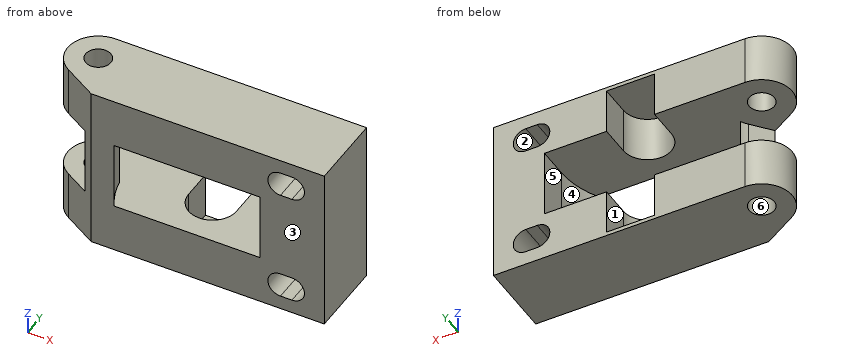
```python
from build123d import *

# Parameters (mm, degrees)
SKETCH1_R               = 1.65
BOSS_EXTRUDE1_DEPTH     = 22
CUT_EXTRUDE1_DEPTH      = 4.5
CUT_EXTRUDE1_DEPTH_BACK = 4.5
CUT_EXTRUDE3_DEPTH      = 10.5
CUT_EXTRUDE3_DEPTH_BACK = 10.5
CUT_EXTRUDE2_DEPTH      = 31.740852298


with BuildPart() as part:
    # Sketch1 → Boss-Extrude1 (new body)
    with BuildSketch(Plane.XY):
        with BuildLine():
            Line((-17, -3.464101615), (-12.607695155, -6))
            Line((-12.607695155, -6), (18, -6))
            Line((18, -6), (18, 4))
            Line((18, 4), (-15, 4))
            ThreePointArc((-15, 4), (-18.863703305, 1.03527618), (-17, -3.464101615))
        make_face()
        with Locations((-15, 0)):
            Circle(SKETCH1_R, mode=Mode.SUBTRACT)
    extrude(amount=BOSS_EXTRUDE1_DEPTH)

    # Sketch2 → Cut-Extrude1 (cut, two sides: drawn at the far end of the back side and taken through both)
    with BuildSketch(Plane.XY.offset(11).offset(-CUT_EXTRUDE1_DEPTH_BACK)):
        with BuildLine():
            Line((-11.706008895, -2.763986722), (-19.3, -11.814152904))
            Line((-19.3, -11.814152904), (-19.3, 11.3))
            Line((-19.3, 11.3), (11.3, 11.3))
            Line((11.3, 11.3), (11.3, 0))
            ThreePointArc((11.3, 0), (0.950789146, -11.259928952), (-11.14, -1.894835085))
            ThreePointArc((-11.14, -1.894835085), (-11.396702437, -2.346539297), (-11.706008895, -2.763986722))
        make_face()
    extrude(amount=CUT_EXTRUDE1_DEPTH + CUT_EXTRUDE1_DEPTH_BACK, mode=Mode.SUBTRACT)

    # Sketch4 → Cut-Extrude3 (cut, two sides: drawn at the far end of the back side and taken through both)
    with BuildSketch(Plane.XY.offset(11).offset(-CUT_EXTRUDE3_DEPTH_BACK)):
        with BuildLine():
            Line((-3.15, 0), (-3.15, 6.453034263))
            Line((-3.15, 6.453034263), (3.15, 6.453034263))
            Line((3.15, 6.453034263), (3.15, 0))
            ThreePointArc((3.15, 0), (0, -3.15), (-3.15, 0))
        make_face()
    extrude(amount=CUT_EXTRUDE3_DEPTH + CUT_EXTRUDE3_DEPTH_BACK, mode=Mode.SUBTRACT)

    # Sketch3 → Cut-Extrude2 (cut, through all)
    with BuildSketch(Plane.XZ.offset(6)):
        with BuildLine():
            Line((13.75, 16.85), (12.25, 16.85))
            ThreePointArc((12.25, 16.85), (10.6, 18.5), (12.25, 20.15))
            Line((12.25, 20.15), (13.75, 20.15))
            ThreePointArc((13.75, 20.15), (15.4, 18.5), (13.75, 16.85))
        make_face()
        with BuildLine():
            Line((13.75, 5.15), (12.25, 5.15))
            ThreePointArc((12.25, 5.15), (10.6, 3.5), (12.25, 1.85))
            Line((12.25, 1.85), (13.75, 1.85))
            ThreePointArc((13.75, 1.85), (15.4, 3.5), (13.75, 5.15))
        make_face()
    extrude(amount=-CUT_EXTRUDE2_DEPTH, mode=Mode.SUBTRACT)


solid = part.part
```
Part model, mm, in its own coordinate system. Face numbers are marked on the shaded views. A direction names the side the tool comes from. Coordinates: 2 decimals unless noted, no trailing zeros. Write each loop counter-clockwise with the first axis right and the second up, starting at its lowest first coordinate (ties: lowest second). Pieces come first, ordered by that corner, then holes.
Item 1: Which spindle directions (+Z, -Z, +X, -X, +Y, -Y) get a long thin tool onto all of the face, cutting with end or side? Do the marked faces 1, 2 and 3. Say none if no direction does.
Item 2: Probe line 1 (X direction, y = 0, z = 3.5); line 2 (Z direction, x = -11, y = 2.5); line 3 (X direction, y = 0, z = 20.25). List the from-to ranges inside material, lowest first.
Item 3: Slice it at B-B (x = -5). Write the cut outline in (y, z).
Item 4: Mould opens along Y. For the marked faces 4, 5 and 6 say: released by +Y, released by -Y, zero draft, split by the parting line, or undercut.
Item 5: Pin check, flat tips, straight feed: pin 1 (1.2 mm diameter, centred on y = 2.5, z = 11, fed in from -X); pin 2 (2 mm diameter, centred on x = -15, y = 0, fed in from +Z); pin 3 (1.2 mm diameter, centred on y = 2.5, z = 3.5, fed in from -X); pin 4 (2 mm diameter, centred on y = 2.5, z = 6.5, fed in from -X). Stop position of each tip, or through.
Item 6: Slice it at A-A (z = 18.5). Write the cut outline in (x, y).
Item 7: Slice it at D-D (y = -2.25). Write the cut outline in (x, z), and give its area (3 significant figures).
Item 8: Slice it at C-C (y = -0.5). Count the separate pieces of the cut face and the enclosed holes in it, and give its area (3 significant figures).
Results found:
1. face 1: +Y
1. face 2: +Y, -Y
1. face 3: +Z, -Z, +X, -X, -Y
2. line 1: x = -19 to -16.65, -13.35 to -3.15, 3.15 to 10.6, 15.4 to 18
2. line 2: z = 0 to 6.5, 15.5 to 22
2. line 3: x = -19 to -16.65, -13.35 to -3.15, 3.15 to 18
3. outline: (-6, 0) - (4, 0) - (4, 6.5) - (-6, 6.5) - close; (-6, 15.5) - (4, 15.5) - (4, 22) - (-6, 22) - close
4. face 4: released by +Y
4. face 5: zero draft
4. face 6: undercut
5. pin 1: stops at x = 11.3
5. pin 2: passes through
5. pin 3: stops at x = -18.52
5. pin 4: stops at x = -18.71
6. outline: (-17, -3.46) - (-12.61, -6) - (10.6, -6) - (10.6, 4) - (3.15, 4) - (3.15, 0) arc R3.15 cw to (-3.15, 0) - (-3.15, 4) - (-15, 4) arc R4 ccw to start; (15.4, -6) - (18, -6) - (18, 4) - (15.4, 4) - close; hole circle Ø3.3 at (-15, 0)
7. outline: (-18.31, 0) - (18, 0) - (18, 22) - (-18.31, 22) - (-18.31, 15.5) - (-11.34, 15.5) - (-11.34, 6.5) - (-18.31, 6.5) - close; hole (-11.07, 6.5) - (-2.2, 6.5) - (-2.2, 0.5) - (2.2, 0.5) - (2.2, 6.5) - (11.07, 6.5) - (11.07, 15.5) - (2.2, 15.5) - (2.2, 21.5) - (-2.2, 21.5) - (-2.2, 15.5) - (-11.07, 15.5) - close; hole (12.25, 1.85) - (13.75, 1.85) arc R1.65 ccw to (13.75, 5.15) - (12.25, 5.15) arc R1.65 ccw to start; hole (12.25, 16.85) - (13.75, 16.85) arc R1.65 ccw to (13.75, 20.15) - (12.25, 20.15) arc R1.65 ccw to start
7. area: 457 mm2
8. separate pieces: 3
8. enclosed holes: 2
8. area: 398 mm2
